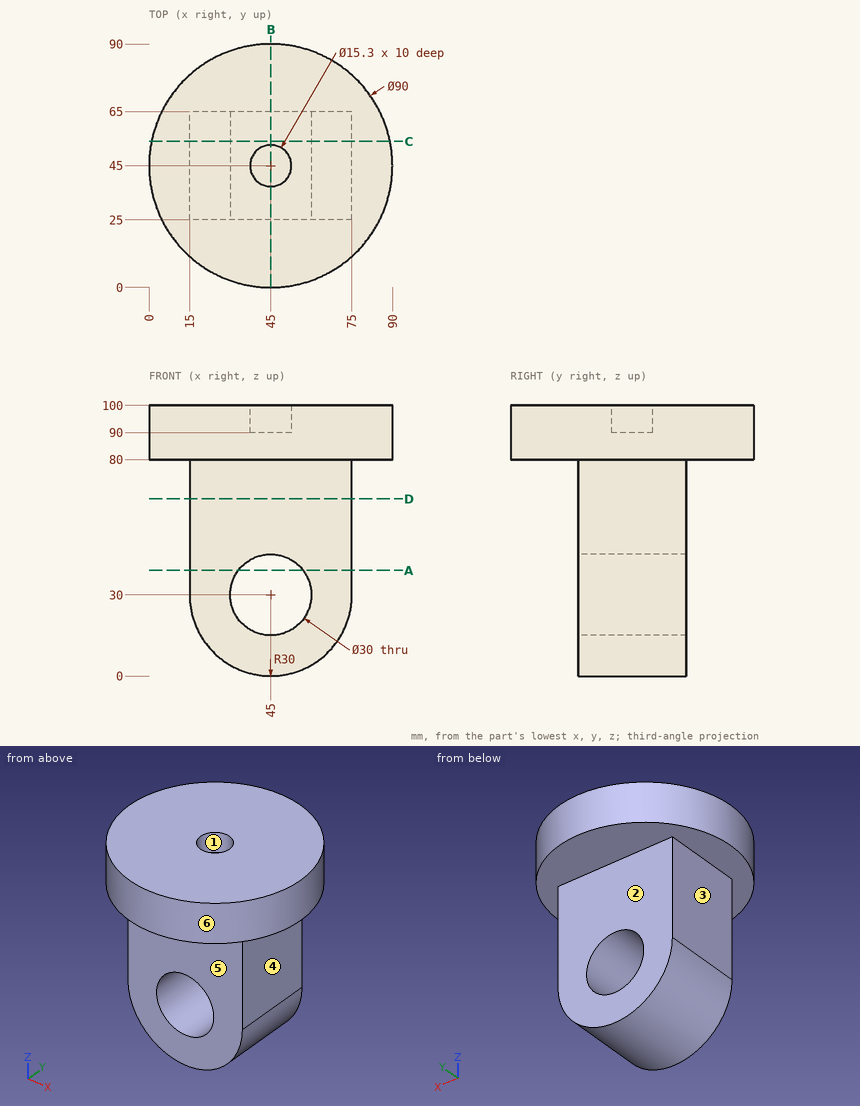
Input: dimensioned drawing with shaded views. Units: mm. Origin: part minimum x, y, z. A direction names the side the tool comes from. Round coordinates to 2 decimals unless told otherwise and drop trailing zeros. Order: outer loops, then holes, each group sorted by start corner. A loop starts at its lowest first (then second) coordinate and runs counter-clockwise, first axis right, second up.
Q1. Access query for the marked faces 4, 5 and 6. Directions: +Z, -Z, +X, -X, +Y, -Y. A direction counts if a zero-diameter tool reaches every point of the face in a straight line with its end or side. Return the directions, or none.
Result sheet:
face 4: -Z, +X, +Y, -Y
face 5: -Z, +X, -X, -Y
face 6: +Z, -Z
Q2. Section D-D, the plane z = 65.5. Output: boundary loops of the cut face in (x, y), and give its area (3 significant figures).
Result sheet:
outline: (15, 25) - (75, 25) - (75, 65) - (15, 65) - close
area: 2,400 mm2
Q3. Mould query, pull axis X, two halves, no side actions, for the marked faces 1, 2 and 3. Classes: released by +X, released by -X, zero draft, split by the parting line, or undercut.
Result sheet:
face 1: undercut
face 2: zero draft
face 3: released by -X
Q4. Section A-A, the plane z = 39. Output: boundary loops of the cut face in (x, y).
Result sheet:
outline: (15, 25) - (33, 25) - (33, 65) - (15, 65) - close; (57, 25) - (75, 25) - (75, 65) - (57, 65) - close
Q5. Material intervals for probe 1 along X at (y, z) = (55.5, 30); probe 2 along Y at (x, z) = (65.5, 41.5); probe 3 along Z at (x, y) = (78, 70), sorted ascending.
Result sheet:
probe 1: x = 15 to 30, 60 to 75
probe 2: y = 25 to 65
probe 3: z = 80 to 100
Q6. Section C-C, the plane y = 54. Output: boundary loops of the cut face in (x, z).
Result sheet:
outline: (0.91, 80) - (15, 80) - (15, 30) arc R30 ccw to (75, 30) - (75, 80) - (89.09, 80) - (89.09, 100) - (0.91, 100) - close; hole circle Ø30 at (45, 30)
Q7. Section B-B, the plane x = 45. Output: boundary loops of the cut face in (y, z), and give its area (3 significant figures).
Result sheet:
outline: (0, 80) - (25, 80) - (25, 45) - (65, 45) - (65, 80) - (90, 80) - (90, 100) - (52.65, 100) - (52.65, 90) - (37.35, 90) - (37.35, 100) - (0, 100) - close; (25, 0) - (65, 0) - (65, 15) - (25, 15) - close
area: 3,650 mm2
Q8. Pin query (flat end, axial travel): pin 1 (1 mm diameter, centred on y = 40, z = 46, fed in from -X); pin 2 (4 mm diameter, centred on x = 26, z = 37.5, fed in from +Y); pin 3 (1 mm diameter, centred on x = 27, y = 27, fed in from -Z); pin 4 (24 mm diameter, centred on x = 45, z = 30, fed in from -Y) (3 decimals). Return the tip coordinate at first contact, or that it passes through.
Result sheet:
pin 1: stops at x = 15
pin 2: stops at y = 65
pin 3: stops at z = 5.63
pin 4: passes through
